from build123d import *

# Parameters (mm, degrees)
SKETCH1_R           = 2.55
BOSS_EXTRUDE2_DEPTH = 3.6
BOSS_EXTRUDE3_START = -3.6
BOSS_EXTRUDE3_DEPTH = 3.6
SKETCH5_R           = 3.05
BOSS_EXTRUDE6_DEPTH = 0.6
FILLET3_R           = 1


with BuildPart() as part:
    # Sketch1 → Boss-Extrude2 (new body)
    with BuildSketch(Plane(origin=(0, 0, 0), x_dir=(1, 0, 0), z_dir=(0, 1, 0))):
        with BuildLine():
            ThreePointArc((3.087277962, -5.973051053), (3.521946978, -6.509464465), (4.123690803, -6.847962431))
            Line((4.123690803, -6.847962431), (4.363885613, -6.697456058))
            ThreePointArc((4.363885613, -6.697456058), (4.321717278, -6.00832738), (4.02858155, -5.38322903))
            ThreePointArc((4.02858155, -5.38322903), (4.185613137, -5.262059175), (4.339002356, -5.136310217))
            ThreePointArc((4.339002356, -5.136310217), (4.882136527, -5.56255167), (5.544116261, -5.758662187))
            Line((5.544116261, -5.758662187), (5.744798067, -5.55848095))
            ThreePointArc((5.744798067, -5.55848095), (5.550341423, -4.896013504), (5.125457751, -4.35181651))
            ThreePointArc((5.125457751, -4.35181651), (5.251589399, -4.198741821), (5.373151055, -4.042013339))
            ThreePointArc((5.373151055, -4.042013339), (5.997515364, -4.336709306), (6.686536579, -4.380598575))
            Line((6.686536579, -4.380598575), (6.837642357, -4.140780396))
            ThreePointArc((6.837642357, -4.140780396), (6.500648273, -3.538193066), (5.965322098, -3.102185738))
            ThreePointArc((5.965322098, -3.102185738), (6.05422904, -2.924882019), (6.137867523, -2.745033035))
            ThreePointArc((6.137867523, -2.745033035), (6.812153737, -2.893406229), (7.493666033, -2.782873458))
            Line((7.493666033, -2.782873458), (7.587618709, -2.515443823))
            ThreePointArc((7.587618709, -2.515443823), (7.124985474, -2.002952854), (6.506060286, -1.696998421))
            ThreePointArc((6.506060286, -1.696998421), (6.553284356, -1.50435642), (6.594805684, -1.310405312))
            ThreePointArc((6.594805684, -1.310405312), (7.285202277, -1.305015683), (7.925031781, -1.045603446))
            Line((7.925031781, -1.045603446), (7.957120175, -0.763972393))
            ThreePointArc((7.957120175, -0.763972393), (7.392046152, -0.367276222), (6.720557445, -0.206716516))
            ThreePointArc((6.720557445, -0.206716516), (6.723730631, -0.008396108), (6.721052751, 0.189931605))
            ThreePointArc((6.721052751, 0.189931605), (7.392940354, 0.3488138), (7.959003343, 0.744097489))
            Line((7.959003343, 0.744097489), (7.927618409, 1.025807803))
            ThreePointArc((7.927618409, 1.025807803), (7.28843877, 1.286817174), (6.598057791, 1.293931018))
            ThreePointArc((6.598057791, 1.293931018), (6.557020976, 1.487985219), (6.510278168, 1.680744559))
            ThreePointArc((6.510278168, 1.680744559), (7.129965532, 1.985152302), (7.593877244, 2.496486269))
            Line((7.593877244, 2.496486269), (7.500592754, 2.764149712))
            ThreePointArc((7.500592754, 2.764149712), (6.819358634, 2.876384183), (6.144703968, 2.729695448))
            ThreePointArc((6.144703968, 2.729695448), (6.061514909, 2.909752755), (5.973051053, 3.087277962))
            ThreePointArc((5.973051053, 3.087277962), (6.509464465, 3.521946978), (6.847962431, 4.123690803))
            Line((6.847962431, 4.123690803), (6.697456058, 4.363885613))
            ThreePointArc((6.697456058, 4.363885613), (6.00832738, 4.321717278), (5.38322903, 4.02858155))
            ThreePointArc((5.38322903, 4.02858155), (5.262059175, 4.185613137), (5.136310217, 4.339002356))
            ThreePointArc((5.136310217, 4.339002356), (5.56255167, 4.882136527), (5.758662187, 5.544116261))
            Line((5.758662187, 5.544116261), (5.55848095, 5.744798067))
            ThreePointArc((5.55848095, 5.744798067), (4.896013504, 5.550341423), (4.35181651, 5.125457751))
            ThreePointArc((4.35181651, 5.125457751), (4.198741821, 5.251589399), (4.042013339, 5.373151055))
            ThreePointArc((4.042013339, 5.373151055), (4.336709306, 5.997515364), (4.380598575, 6.686536579))
            Line((4.380598575, 6.686536579), (4.140780396, 6.837642357))
            ThreePointArc((4.140780396, 6.837642357), (3.538193066, 6.500648273), (3.102185738, 5.965322098))
            ThreePointArc((3.102185738, 5.965322098), (2.924882019, 6.05422904), (2.745033035, 6.137867523))
            ThreePointArc((2.745033035, 6.137867523), (2.893406229, 6.812153737), (2.782873458, 7.493666033))
            Line((2.782873458, 7.493666033), (2.515443823, 7.587618709))
            ThreePointArc((2.515443823, 7.587618709), (2.002952854, 7.124985474), (1.696998421, 6.506060286))
            ThreePointArc((1.696998421, 6.506060286), (1.50435642, 6.553284356), (1.310405312, 6.594805684))
            ThreePointArc((1.310405312, 6.594805684), (1.305015683, 7.285202277), (1.045603446, 7.925031781))
            Line((1.045603446, 7.925031781), (0.763972393, 7.957120175))
            ThreePointArc((0.763972393, 7.957120175), (0.367276222, 7.392046152), (0.206716516, 6.720557445))
            ThreePointArc((0.206716516, 6.720557445), (0.008396108, 6.723730631), (-0.189931605, 6.721052751))
            ThreePointArc((-0.189931605, 6.721052751), (-0.3488138, 7.392940354), (-0.744097489, 7.959003343))
            Line((-0.744097489, 7.959003343), (-1.025807803, 7.927618409))
            ThreePointArc((-1.025807803, 7.927618409), (-1.286817174, 7.28843877), (-1.293931018, 6.598057791))
            ThreePointArc((-1.293931018, 6.598057791), (-1.487985219, 6.557020976), (-1.680744559, 6.510278168))
            ThreePointArc((-1.680744559, 6.510278168), (-1.985152302, 7.129965532), (-2.496486269, 7.593877244))
            Line((-2.496486269, 7.593877244), (-2.764149712, 7.500592754))
            ThreePointArc((-2.764149712, 7.500592754), (-2.876384183, 6.819358634), (-2.729695448, 6.144703968))
            ThreePointArc((-2.729695448, 6.144703968), (-2.909752755, 6.061514909), (-3.087277962, 5.973051053))
            ThreePointArc((-3.087277962, 5.973051053), (-3.521946978, 6.509464465), (-4.123690803, 6.847962431))
            Line((-4.123690803, 6.847962431), (-4.363885613, 6.697456058))
            ThreePointArc((-4.363885613, 6.697456058), (-4.321717278, 6.00832738), (-4.02858155, 5.38322903))
            ThreePointArc((-4.02858155, 5.38322903), (-4.185613137, 5.262059175), (-4.339002356, 5.136310217))
            ThreePointArc((-4.339002356, 5.136310217), (-4.882136527, 5.56255167), (-5.544116261, 5.758662187))
            Line((-5.544116261, 5.758662187), (-5.744798067, 5.55848095))
            ThreePointArc((-5.744798067, 5.55848095), (-5.550341423, 4.896013504), (-5.125457751, 4.35181651))
            ThreePointArc((-5.125457751, 4.35181651), (-5.251589399, 4.198741821), (-5.373151055, 4.042013339))
            ThreePointArc((-5.373151055, 4.042013339), (-5.997515364, 4.336709306), (-6.686536579, 4.380598575))
            Line((-6.686536579, 4.380598575), (-6.837642357, 4.140780396))
            ThreePointArc((-6.837642357, 4.140780396), (-6.500648273, 3.538193066), (-5.965322098, 3.102185738))
            ThreePointArc((-5.965322098, 3.102185738), (-6.05422904, 2.924882019), (-6.137867523, 2.745033035))
            ThreePointArc((-6.137867523, 2.745033035), (-6.812153737, 2.893406229), (-7.493666033, 2.782873458))
            Line((-7.493666033, 2.782873458), (-7.587618709, 2.515443823))
            ThreePointArc((-7.587618709, 2.515443823), (-7.124985474, 2.002952854), (-6.506060286, 1.696998421))
            ThreePointArc((-6.506060286, 1.696998421), (-6.553284356, 1.50435642), (-6.594805684, 1.310405312))
            ThreePointArc((-6.594805684, 1.310405312), (-7.285202277, 1.305015683), (-7.925031781, 1.045603446))
            Line((-7.925031781, 1.045603446), (-7.957120175, 0.763972393))
            ThreePointArc((-7.957120175, 0.763972393), (-7.392046152, 0.367276222), (-6.720557445, 0.206716516))
            ThreePointArc((-6.720557445, 0.206716516), (-6.723730631, 0.008396108), (-6.721052751, -0.189931605))
            ThreePointArc((-6.721052751, -0.189931605), (-7.392940354, -0.3488138), (-7.959003343, -0.744097489))
            Line((-7.959003343, -0.744097489), (-7.927618409, -1.025807803))
            ThreePointArc((-7.927618409, -1.025807803), (-7.28843877, -1.286817174), (-6.598057791, -1.293931018))
            ThreePointArc((-6.598057791, -1.293931018), (-6.557020976, -1.487985219), (-6.510278168, -1.680744559))
            ThreePointArc((-6.510278168, -1.680744559), (-7.129965532, -1.985152302), (-7.593877244, -2.496486269))
            Line((-7.593877244, -2.496486269), (-7.500592754, -2.764149712))
            ThreePointArc((-7.500592754, -2.764149712), (-6.819358634, -2.876384183), (-6.144703968, -2.729695448))
            ThreePointArc((-6.144703968, -2.729695448), (-6.061514909, -2.909752755), (-5.973051053, -3.087277962))
            ThreePointArc((-5.973051053, -3.087277962), (-6.509464465, -3.521946978), (-6.847962431, -4.123690803))
            Line((-6.847962431, -4.123690803), (-6.697456058, -4.363885613))
            ThreePointArc((-6.697456058, -4.363885613), (-6.00832738, -4.321717278), (-5.38322903, -4.02858155))
            ThreePointArc((-5.38322903, -4.02858155), (-5.262059175, -4.185613137), (-5.136310217, -4.339002356))
            ThreePointArc((-5.136310217, -4.339002356), (-5.56255167, -4.882136527), (-5.758662187, -5.544116261))
            Line((-5.758662187, -5.544116261), (-5.55848095, -5.744798067))
            ThreePointArc((-5.55848095, -5.744798067), (-4.896013504, -5.550341423), (-4.35181651, -5.125457751))
            ThreePointArc((-4.35181651, -5.125457751), (-4.198741821, -5.251589399), (-4.042013339, -5.373151055))
            ThreePointArc((-4.042013339, -5.373151055), (-4.336709306, -5.997515364), (-4.380598575, -6.686536579))
            Line((-4.380598575, -6.686536579), (-4.140780396, -6.837642357))
            ThreePointArc((-4.140780396, -6.837642357), (-3.538193066, -6.500648273), (-3.102185738, -5.965322098))
            ThreePointArc((-3.102185738, -5.965322098), (-2.924882019, -6.05422904), (-2.745033035, -6.137867523))
            ThreePointArc((-2.745033035, -6.137867523), (-2.893406229, -6.812153737), (-2.782873458, -7.493666033))
            Line((-2.782873458, -7.493666033), (-2.515443823, -7.587618709))
            ThreePointArc((-2.515443823, -7.587618709), (-2.002952854, -7.124985474), (-1.696998421, -6.506060286))
            ThreePointArc((-1.696998421, -6.506060286), (-1.50435642, -6.553284356), (-1.310405312, -6.594805684))
            ThreePointArc((-1.310405312, -6.594805684), (-1.305015683, -7.285202277), (-1.045603446, -7.925031781))
            Line((-1.045603446, -7.925031781), (-0.763972393, -7.957120175))
            ThreePointArc((-0.763972393, -7.957120175), (-0.367276222, -7.392046152), (-0.206716516, -6.720557445))
            ThreePointArc((-0.206716516, -6.720557445), (-0.008396108, -6.723730631), (0.189931605, -6.721052751))
            ThreePointArc((0.189931605, -6.721052751), (0.3488138, -7.392940354), (0.744097489, -7.959003343))
            Line((0.744097489, -7.959003343), (1.025807803, -7.927618409))
            ThreePointArc((1.025807803, -7.927618409), (1.286817174, -7.28843877), (1.293931018, -6.598057791))
            ThreePointArc((1.293931018, -6.598057791), (1.487985219, -6.557020976), (1.680744559, -6.510278168))
            ThreePointArc((1.680744559, -6.510278168), (1.985152302, -7.129965532), (2.496486269, -7.593877244))
            Line((2.496486269, -7.593877244), (2.764149712, -7.500592754))
            ThreePointArc((2.764149712, -7.500592754), (2.876384183, -6.819358634), (2.729695448, -6.144703968))
            ThreePointArc((2.729695448, -6.144703968), (2.909752755, -6.061514909), (3.087277962, -5.973051053))
        make_face()
        with Locations(Location((0, 0, 0), (0, 0, 270))):
            Circle(SKETCH1_R, mode=Mode.SUBTRACT)
    extrude(amount=BOSS_EXTRUDE2_DEPTH)

    # Sketch2 → Boss-Extrude3 (add)
    with BuildSketch(Plane(origin=(0, 3.6, 0), x_dir=(1, 0, 0), z_dir=(0, 1, 0)).offset(BOSS_EXTRUDE3_START)):
        with BuildLine():
            Line((-1.900657781, -1.7), (1.900657781, -1.7))
            ThreePointArc((1.900657781, -1.7), (0, -2.55), (-1.900657781, -1.7))
        make_face()
    extrude(amount=BOSS_EXTRUDE3_DEPTH)

    # Sketch5 → Boss-Extrude6 (add)
    with BuildSketch(Plane(origin=(0, 3.6, 0), x_dir=(1, 0, 0), z_dir=(0, 1, 0))):
        with Locations(Location((0, 0, 0), (0, 0, 270))):
            Circle(SKETCH5_R)
        with BuildLine():
            Line((1.900657781, -1.7), (-1.900657781, -1.7))
            ThreePointArc((-1.900657781, -1.7), (0, 2.55), (1.900657781, -1.7))
        make_face(mode=Mode.SUBTRACT)
    extrude(amount=BOSS_EXTRUDE6_DEPTH)

    # Fillet3
    # the kernel refuses this fillet: 1 mm, written as the material it adds along each edge
    with BuildSketch(Plane(origin=(0, 3.6, 0), x_dir=(0, 0, 1), z_dir=(-1, 0, 0))) as fillet3_piece_1:
        with BuildLine():
            CenterArc((3.966515139, 1), FILLET3_R, 203.578178478, 66.421821522)
            Line((3.05, 0.6), (3.031669697, 0.592))
            ThreePointArc((3.031669697, 0.592), (3.03, 0.3), (3.03, 0))
            Line((3.03, 0), (3.05, -0.02))
            Line((3.05, -0.02), (3.966515139, -0.02))
            Line((3.966515139, -0.02), (3.966515139, 0))
        make_face()
    revolve(axis=Axis((0, 3.6, 0), (0, 1, 0)))


solid = part.part
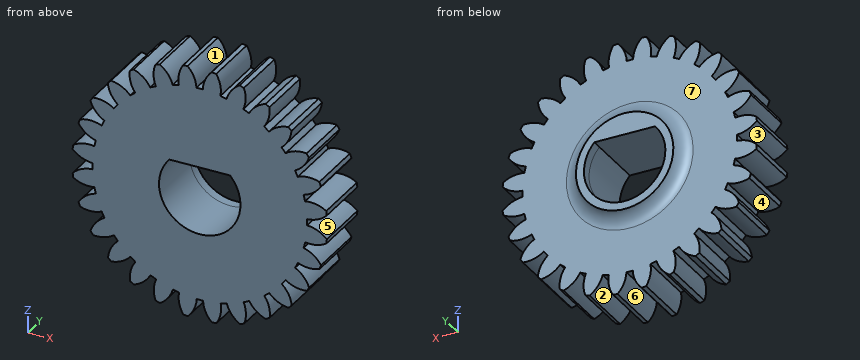
Work out the finished part from the listing and answer in its coordinate system (mm). Face numbers are marked on the shaded views. A direction names the side the tool comes from. Round coordinates to 2 decimals unless told otherwise and drop trailing zeros. Order: outer loops, then holes, each group sorted by start corner. A loop starts at its lowest first (then second) coordinate and runs counter-clockwise, first axis right, second up. Notation, with made-up numbers: M 77,83 L 91,83 A23 cw 91,110 Z; hole C 15.25,-7 d1. An arc over 180 degrees is marked long. One line per item, written item: value.
Q1. Find section B-B on x = 0. Write down the section's boundary in (y, z), then the cut area to 3 significant figures.
Derived:
outline: M 0,-6.72 L 3.6,-6.72 L 3.6,-3.97 A1 cw 4.2,-3.05 L 4.2,-2.55 L 0,-2.55 Z; M 0,1.7 L 4.2,1.7 L 4.2,3.05 A1 cw 3.6,3.97 L 3.6,6.72 L 0,6.72 Z
area: 34.5 mm²
Q2. Find section C-C on y = 3.9. Write down the section's boundary in (x, z).
Derived:
outline: C 0,0 d6.5; hole M -1.9,1.7 A2.55 ccw long 1.9,1.7 Z
Q3. Find section A-A on z = 0. Write down the section's boundary in (x, y).
Derived:
outline: M -6.72,0 L -2.55,0 L -2.55,4.2 L -3.05,4.2 A1 cw -3.97,3.6 L -6.72,3.6 Z; M 2.55,0 L 6.72,0 L 6.72,3.6 L 3.97,3.6 A1 cw 3.05,4.2 L 2.55,4.2 Z
Q4. Determine the mould class of the marked faces 5, 6 and 7 for opening direction Z: released by +Z, released by -Z, zero draft, split by the parting line, or undercut.
Derived:
face 5: undercut
face 6: released by -Z
face 7: zero draft
Q5. For the marked faces 1, 2, 3 and 4, determine the directions among +Z, -Z, +X, -X, +Y, -Y from which every point of the face is accessible in a straight line to the end or side of a thin tool.
Derived:
face 1: +Z, +Y, -Y
face 2: -Z, +Y, -Y
face 3: -X, +Y, -Y
face 4: +Y, -Y
Q6. Straight lines are drawn through the part: line 1 (X direction, y = 2.7, z = 0); line 2 (Z direction, x = 0, y = 1.3); line 3 (X direction, y = 1.4, z = 6.25). For each, find the intervals that lie inside material, in ascending order.
Derived:
line 1: -6.72 to -2.55, 2.55 to 6.72
line 2: -6.72 to -2.55, 1.7 to 6.72
line 3: -4.38 to -3.29, -2.79 to 2.77, 3.27 to 4.37
Q7. Flat-ended cylindrical pins translate along their axes: pin 1 (2 mm diameter, centred on x = 4, y = 0.5, fed in from -Z); pin 2 (1 mm diameter, centred on y = 2, z = 5, fed in from +X). Find the tip coordinate at first contact, or state that the pin passes through.
Derived:
pin 1: z = -6.84
pin 2: x = 5.74
